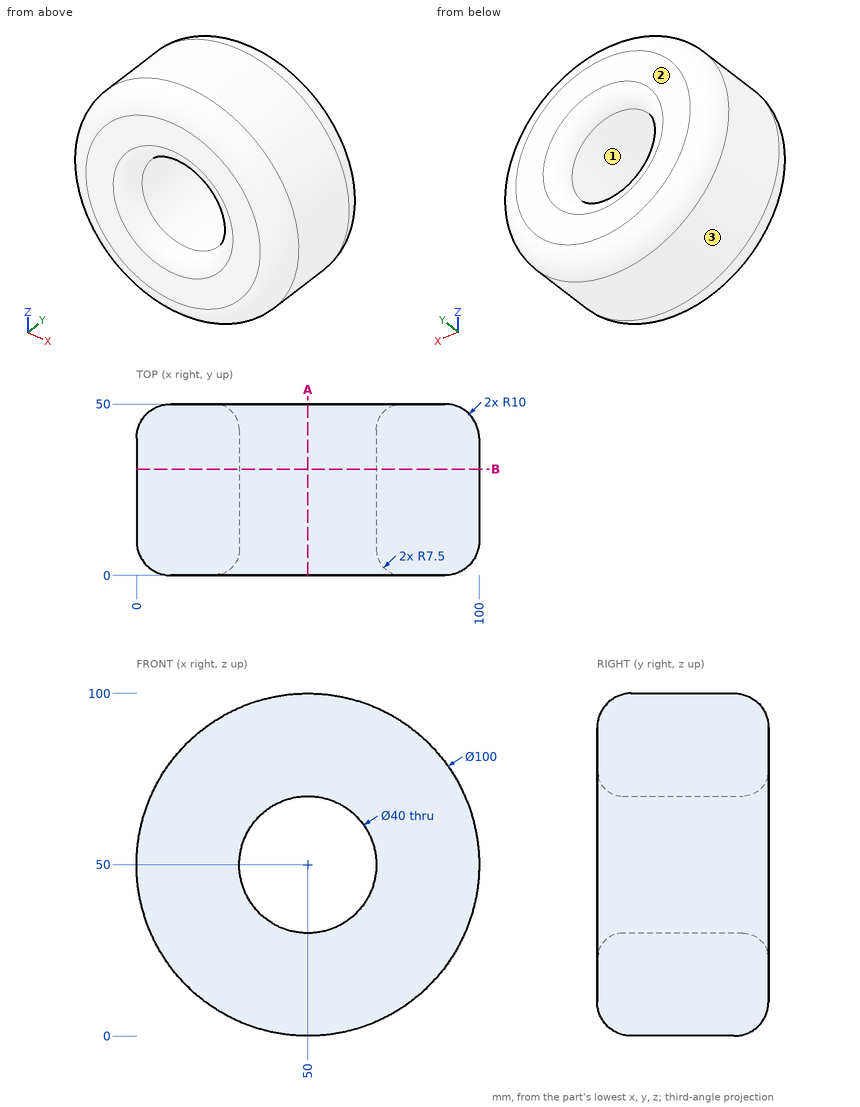
The figure shows three views and two pictorial views of one solid part (mm, origin at its lowest corner). Answer the questions. Give positions to 0.01 mm unless a question says otherwise; leave off trailing zeros. Order: outer loops, then holes, each group sorted by start corner. A loop starts at its lowest first (then second) coordinate and runs counter-clockwise, first axis right, second up. Notation, with made-up numbers: (22, 43) -> (50, 43) arc R26 cw to (50, 65) -> close; hole circle Ø6 at (68.25, -17). An arc over 180 degrees is marked (long way). Answer as CSV lines item,"result". Start each with the question number.
(1) Consider line 1 along X through (y, z) = (29.5, 50); line 2 along Y through (x, z) = (38.5, 74.5); line 3 along Z through (x, y) = (65, 34.5). Determine where each line is inside the solid, lowest interval first.
(2) Each of these flat-tipped pins is pushed along its axis until it touches: pin 1 Ø1.5 at (y, z) = (14.5, 88) entering from +X; pin 2 Ø2 at (x, z) = (35.5, 30) entering from +Y; pin 3 Ø8 at (x, y) = (55, 11.5) entering from -Z. Where does it stop, or does it pass through?
(3) For a pull along Z with two mould halves and no side action, classify the marked faces 1, 2 and 3 as released by +Z, released by -Z, zero draft, split by the parting line, or undercut.
(4) Section B-B, the plane y = 31 is taken. Write down the section's boundary in (x, z).
(5) Section A-A, the plane x = 50 is taken. Write down the section's boundary in (y, z).
Entries:
1,line 1,"0 to 30, 70 to 100"
1,line 2,"0.01 to 49.99"
1,line 3,"2.3 to 36.77, 63.23 to 97.7"
2,pin 1,"x = 83.35"
2,pin 2,"y = 49.78"
2,pin 3,"z = 0.01"
3,face 1,"undercut"
3,face 2,"zero draft"
3,face 3,"split by the parting line"
4,outline,"circle Ø100 at (50, 50); hole circle Ø40 at (50, 50)"
5,outline,"(0, 10) arc R10 ccw to (10, 0) -> (40, 0) arc R10 ccw to (50, 10) -> (50, 22.5) arc R7.5 ccw to (42.5, 30) -> (7.5, 30) arc R7.5 ccw to (0, 22.5) -> close; (0, 77.5) arc R7.5 ccw to (7.5, 70) -> (42.5, 70) arc R7.5 ccw to (50, 77.5) -> (50, 90) arc R10 ccw to (40, 100) -> (10, 100) arc R10 ccw to (0, 90) -> close"
